Autodesk Inventor part; units mm, degrees
ref_plane "YZ Plane" through (0, 0, 0) normal (1, 0, 0) x (0, 1, 0)
ref_plane "XZ Plane" through (0, 0, 0) normal (0, 1, 0) x (-1, 0, 0)
ref_plane "XY Plane" through (0, 0, 0) normal (0, 0, 1) x (1, 0, 0)
sketch "Boceto1" plane through (0, 0, 0) normal (0, 0, 1) x (1, 0, 0)
  line L0 (0, 55.8594) -> (0, -55.8594) construction
  line L1 (110.1563, 0) -> (-110.1563, 0) construction
  line L2 (-4.5, 41.4844) -> (4.5, 41.4844)
  line L3 (4.5, 41.4844) -> (4.5, -48.5156)
  line L4 (4.5, -48.5156) -> (-4.5, -48.5156)
  line L5 (-4.5, -48.5156) -> (-4.5, 41.4844)
  arc A0 (-4.5, -48.5156) -> (4.5, -48.5156) centre (0, -48.5156) ccw
  circle A1 centre (0, -48.5156) radius 2.5
  point P0 (0, 0)
  point P1 (0, 0)
  point P2 (0, 41.4844)
  point P3 (0, -12.5156)
  point P4 (0, -48.5156)
  dimension "d0" = 90
  dimension "d1" = 9
  dimension "d2" = 4.5
  dimension "d3" = 5
  dimension "d4" = 36
  dimension "d5" = 41.4844
  dimension "d6" = 105.6563
  dimension "d7" = 55.8594
extrude "Extrusión1" add sketch "Boceto1" against normal blind 4 contours L2 L3 L4 A1 L5 | L4 A1 A0
hole "Agujero1" at (0, -12.5156, 0) direction (0, 0, -1) diameter 4 end through all
properties part number "1-HUDSON-8-33-TDR HAND PUMP HANDLE"
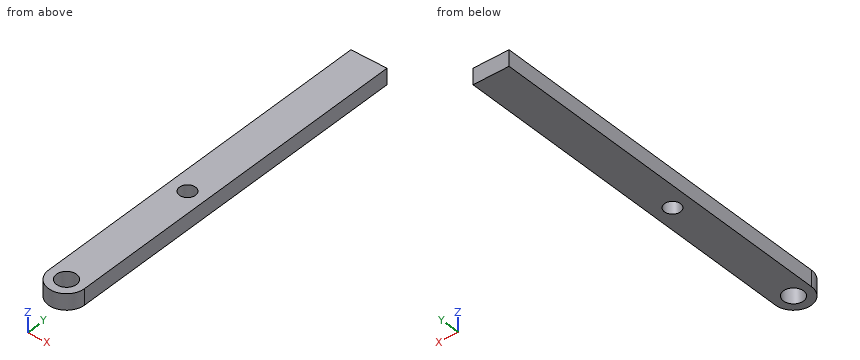
Source: CAD feature listing. Evaluate the final solid. Frame: model axes, mm. Coordinates: 2 decimals unless noted, no trailing zeros. Loops run counter-clockwise (first coordinate to the right, second up) from the corner with the lowest first, then second, coordinate; pieces in that order, holes last. Notation, with made-up numbers: (76.25, -39) -> (112.25, -39) arc R19 cw to (112.25, -12) -> close; hole circle Ø2 at (32, 45.5). An arc over 180 degrees is marked (long way). One line per item, written item: value. Start each with the question number.
Q1. Contact query for a flat-ended pin moving along its axis: P1, Ø4, axis at x = -1.5, y = -31.5, coming from the +Z side. Output: stop coordinate, or through.
Q2. Section query B-B, the plane z = -0.8. Return the cut outline in (x, y).
Q3. Section query A-A, the plane x = 0. Return the cut outline in (y, z).
Q4. Line query: line 1 along Y through (x, z) = (0, -2); line 2 along X through (y, z) = (-47, -3.8); line 3 along Y through (x, z) = (3.75, -0.45). Output: solid intervals per line, ascending.
Results:
1. P1: z = 0
2. outline: (-4.5, -48.52) arc R4.5 ccw to (4.5, -48.52) -> (4.5, 41.48) -> (-4.5, 41.48) -> close; hole circle Ø5 at (0, -48.52); hole circle Ø4 at (0, -12.52)
3. outline: (-53.02, -4) -> (-51.02, -4) -> (-51.02, 0) -> (-53.02, 0) -> close; (-46.02, -4) -> (-14.52, -4) -> (-14.52, 0) -> (-46.02, 0) -> close; (-10.52, -4) -> (41.48, -4) -> (41.48, 0) -> (-10.52, 0) -> close
4. line 1: -53.02 to -51.02, -46.02 to -14.52, -10.52 to 41.48
4. line 2: -4.5 to -1.99, 1.99 to 4.5
4. line 3: -51 to 41.48
